Part model, mm, in its own coordinate system. A direction names the side the tool comes from. Round coordinates to 2 decimals unless told otherwise and drop trailing zeros. Loops run counter-clockwise (first coordinate to the right, second up) from the corner with the lowest first, then second, coordinate; pieces in that order, holes last.
(1) Flat gauge pins, fed straight in: pin 1 (2 mm diameter, centred on x = 31.5, y = 6.5, fed in from -Z); pin 2 (2 mm diameter, centred on y = 2, z = -3.5, fed in from +X); pin 3 (3.5 mm diameter, centred on y = 4.5, z = -5, fed in from -X). Where does each tip first touch, or does it go through?
(2) Cut at B-B on y = 5.75. List the corners of the cut face in (x, z), then the cut area to 3 significant figures.
(3) Probe probe 1 along X at (y, z) = (2.5, -2.5); probe 2 along Z at (x, y) = (-25, -2.75); probe 3 along X at (y, z) = (4.25, 1). List the from-to ranges inside material, lowest first.
(4) Cut at C-C on x = 11.5. List the corners of the cut face in (y, z), then the cut area to 3 significant figures.
(5) Tool access for faces 1 (the face through (-37.78, 12.75, -3.45)), 2 (the face through (-34.5, 4, -3)), 3 (the face through (41.2, 4, -3)), 4 (the face through (-17.682, 3.576, 1.479)), 5 (the face through (-37.924, -3.947, -3.451)): list every direction of +Z, -Z, +X, -X, +Y, -Y with a clear straight run to the whole face (end or side of a thin tool).
(6) Cut at A-A on z = -1.5. List the corners of the cut face in (x, y).
(7) Cut at D-D on x = -13. List the corners of the cut face in (y, z), then the cut area to 3 significant figures.
from build123d import *

# Parameters (mm, degrees)
BOSS_EXTRUDE1_DEPTH = 3
BOSS_EXTRUDE2_DEPTH = 7


with BuildPart() as part:
    # Sketch1 → Boss-Extrude1 (new body)
    with BuildSketch(Plane.XY):
        with BuildLine():
            ThreePointArc((-43.2, -9.751954051), (-41.735533906, -13.287487956), (-38.2, -14.751954051))
            Line((-38.2, -14.751954051), (38.2, -14.751954051))
            ThreePointArc((38.2, -14.751954051), (41.735533906, -13.287487956), (43.2, -9.751954051))
            Line((43.2, -9.751954051), (43.2, 9.751954051))
            ThreePointArc((43.2, 9.751954051), (41.735533906, 13.287487956), (38.2, 14.751954051))
            Line((38.2, 14.751954051), (35.865969403, 14.751954051))
            Line((35.865969403, 14.751954051), (0, -7.291716438))
            Line((0, -7.291716438), (-35.865969403, 14.751954051))
            Line((-35.865969403, 14.751954051), (-38.2, 14.751954051))
            ThreePointArc((-38.2, 14.751954051), (-41.735533906, 13.287487956), (-43.2, 9.751954051))
            Line((-43.2, 9.751954051), (-43.2, -9.751954051))
        make_face()
        with BuildLine():
            ThreePointArc((-41.2, 9.401954051), (-37.85, 12.751954051), (-34.5, 9.401954051))
            Line((-34.5, 9.401954051), (-34.5, -0.598045949))
            ThreePointArc((-34.5, -0.598045949), (-37.85, -3.948045949), (-41.2, -0.598045949))
            Line((-41.2, -0.598045949), (-41.2, 9.401954051))
        make_face(mode=Mode.SUBTRACT)
        with BuildLine():
            ThreePointArc((34.5, 9.401954051), (37.85, 12.751954051), (41.2, 9.401954051))
            Line((41.2, 9.401954051), (41.2, -0.598045949))
            ThreePointArc((41.2, -0.598045949), (37.85, -3.948045949), (34.5, -0.598045949))
            Line((34.5, -0.598045949), (34.5, 9.401954051))
        make_face(mode=Mode.SUBTRACT)
        with BuildLine():
            Line((34.5, 9.401954051), (34.5, -0.598045949))
            ThreePointArc((34.5, -0.598045949), (37.85, -3.948045949), (41.2, -0.598045949))
            Line((41.2, -0.598045949), (41.2, 9.401954051))
            ThreePointArc((41.2, 9.401954051), (37.85, 12.751954051), (34.5, 9.401954051))
        make_face()
        with BuildLine():
            Line((-41.2, 9.401954051), (-41.2, -0.598045949))
            ThreePointArc((-41.2, -0.598045949), (-37.85, -3.948045949), (-34.5, -0.598045949))
            Line((-34.5, -0.598045949), (-34.5, 9.401954051))
            ThreePointArc((-34.5, 9.401954051), (-37.85, 12.751954051), (-41.2, 9.401954051))
        make_face()
    extrude(amount=BOSS_EXTRUDE1_DEPTH)

    # Sketch1_3 → Boss-Extrude2 (add)
    with BuildSketch(Plane.XY):
        with BuildLine():
            Line((34.5, 9.401954051), (34.5, -0.598045949))
            ThreePointArc((34.5, -0.598045949), (37.85, -3.948045949), (41.2, -0.598045949))
            Line((41.2, -0.598045949), (41.2, 9.401954051))
            ThreePointArc((41.2, 9.401954051), (37.85, 12.751954051), (34.5, 9.401954051))
        make_face()
        with BuildLine():
            Line((-41.2, 9.401954051), (-41.2, -0.598045949))
            ThreePointArc((-41.2, -0.598045949), (-37.85, -3.948045949), (-34.5, -0.598045949))
            Line((-34.5, -0.598045949), (-34.5, 9.401954051))
            ThreePointArc((-34.5, 9.401954051), (-37.85, 12.751954051), (-41.2, 9.401954051))
        make_face()
    extrude(amount=-BOSS_EXTRUDE2_DEPTH)


solid = part.part
Final values:
1. pin 1: stops at z = 0
1. pin 2: stops at x = 41.2
1. pin 3: stops at x = -41.2
2. outline: (-43.2, 0) - (-41.2, 0) - (-41.2, -7) - (-34.5, -7) - (-34.5, 0) - (-21.22, 0) - (-21.22, 3) - (-43.2, 3) - close; (21.22, 0) - (34.5, 0) - (34.5, -7) - (41.2, -7) - (41.2, 0) - (43.2, 0) - (43.2, 3) - (21.22, 3) - close
2. area: 226 mm2
3. probe 1: x = -41.2 to -34.5, 34.5 to 41.2
3. probe 2: z = 0 to 3
3. probe 3: x = -43.2 to -18.78, 18.78 to 43.2
4. outline: (-14.75, 0) - (-0.22, 0) - (-0.22, 3) - (-14.75, 3) - close
4. area: 43.6 mm2
5. face 1: -Z, +Y
5. face 2: -Z, +Y, -Y
5. face 3: -Z, +X, +Y, -Y
5. face 4: +Z, -Z, +Y
5. face 5: -Z, -Y
6. outline: (-41.2, -0.6) arc R3.35 ccw to (-34.5, -0.6) - (-34.5, 9.4) arc R3.35 ccw to (-41.2, 9.4) - close; (34.5, -0.6) arc R3.35 ccw to (41.2, -0.6) - (41.2, 9.4) arc R3.35 ccw to (34.5, 9.4) - close
7. outline: (-14.75, 0) - (0.7, 0) - (0.7, 3) - (-14.75, 3) - close
7. area: 46.4 mm2
